from build123d import *


with BuildPart() as f2:
    # F2: sweep along a path in F1
    with BuildLine(Plane.XZ) as f2_path:
        Line((0, 0), (-0.868731, 2.386819))
    # F0 (on Top) → F2 (sweep)
    with BuildSketch(Plane.XY):
        with BuildLine():
            Line((0, 14.836045), (-1.27, 12.63634))
            ThreePointArc((-1.27, 12.63634), (-1.591732, 12.599857), (-1.912429, 12.555183))
            Line((-1.912429, 12.555183), (-3.689574, 14.369943))
            Line((-3.689574, 14.369943), (-4.372631, 11.92351))
            ThreePointArc((-4.372631, 11.92351), (-4.675182, 11.808161), (-4.974694, 11.685137))
            Line((-4.974694, 11.685137), (-7.147319, 13.000925))
            Line((-7.147319, 13.000925), (-7.200513, 10.461482))
            ThreePointArc((-7.200513, 10.461482), (-7.464873, 10.274516), (-7.72438, 10.080871))
            Line((-7.72438, 10.080871), (-10.155972, 10.815011))
            Line((-10.155972, 10.815011), (-9.57596, 8.342121))
            ThreePointArc((-9.57596, 8.342121), (-9.785518, 8.095285), (-9.988715, 7.843186))
            Line((-9.988715, 7.843186), (-12.526487, 7.94955))
            Line((-12.526487, 7.94955), (-11.349715, 5.698593))
            ThreePointArc((-11.349715, 5.698593), (-11.491304, 5.407397), (-11.625422, 5.112686))
            Line((-11.625422, 5.112686), (-14.109917, 4.58459))
            Line((-14.109917, 4.58459), (-12.410326, 2.697002))
            ThreePointArc((-12.410326, 2.697002), (-12.475048, 2.379743), (-12.531662, 2.060936))
            Line((-12.531662, 2.060936), (-14.806769, 0.931563))
            Line((-14.806769, 0.931563), (-12.691149, -0.474052))
            ThreePointArc((-12.691149, -0.474052), (-12.674939, -0.79744), (-12.65049, -1.120309))
            Line((-12.65049, -1.120309), (-14.573258, -2.779998))
            Line((-14.573258, -2.779998), (-12.174542, -3.615319))
            ThreePointArc((-12.174542, -3.615319), (-12.078418, -3.924516), (-11.974442, -4.231162))
            Line((-11.974442, -4.231162), (-13.424055, -6.316881))
            Line((-13.424055, -6.316881), (-10.892963, -6.529422))
            ThreePointArc((-10.892963, -6.529422), (-10.722965, -6.805), (-10.545996, -7.076155))
            Line((-10.545996, -7.076155), (-11.431369, -9.456851))
            Line((-11.431369, -9.456851), (-8.926939, -9.033258))
            ThreePointArc((-8.926939, -9.033258), (-8.693748, -9.257902), (-8.454906, -9.476527))
            Line((-8.454906, -9.476527), (-8.720408, -12.002613))
            Line((-8.720408, -12.002613), (-6.400003, -10.969501))
            ThreePointArc((-6.400003, -10.969501), (-6.118272, -11.129095), (-5.832563, -11.281454))
            Line((-5.832563, -11.281454), (-5.461512, -13.794206))
            Line((-5.461512, -13.794206), (-3.470931, -12.21649))
            ThreePointArc((-3.470931, -12.21649), (-3.158362, -12.301006), (-2.843739, -12.377526))
            Line((-2.843739, -12.377526), (-1.859449, -14.719058))
            Line((-1.859449, -14.719058), (-0.323768, -12.695872))
            ThreePointArc((-0.323768, -12.695872), (0, -12.7), (0.323768, -12.695872))
            Line((0.323768, -12.695872), (1.859449, -14.719058))
            Line((1.859449, -14.719058), (2.843739, -12.377526))
            ThreePointArc((2.843739, -12.377526), (3.158362, -12.301006), (3.470931, -12.21649))
            Line((3.470931, -12.21649), (5.461512, -13.794206))
            Line((5.461512, -13.794206), (5.832563, -11.281454))
            ThreePointArc((5.832563, -11.281454), (6.118272, -11.129095), (6.400003, -10.969501))
            Line((6.400003, -10.969501), (8.720408, -12.002613))
            Line((8.720408, -12.002613), (8.454906, -9.476527))
            ThreePointArc((8.454906, -9.476527), (8.693748, -9.257902), (8.926939, -9.033258))
            Line((8.926939, -9.033258), (11.431369, -9.456851))
            Line((11.431369, -9.456851), (10.545996, -7.076155))
            ThreePointArc((10.545996, -7.076155), (10.722965, -6.805), (10.892963, -6.529422))
            Line((10.892963, -6.529422), (13.424055, -6.316881))
            Line((13.424055, -6.316881), (11.974442, -4.231162))
            ThreePointArc((11.974442, -4.231162), (12.078418, -3.924516), (12.174542, -3.615319))
            Line((12.174542, -3.615319), (14.573258, -2.779998))
            Line((14.573258, -2.779998), (12.65049, -1.120309))
            ThreePointArc((12.65049, -1.120309), (12.674939, -0.79744), (12.691149, -0.474052))
            Line((12.691149, -0.474052), (14.806769, 0.931563))
            Line((14.806769, 0.931563), (12.531662, 2.060936))
            ThreePointArc((12.531662, 2.060936), (12.475048, 2.379743), (12.410326, 2.697002))
            Line((12.410326, 2.697002), (14.109917, 4.58459))
            Line((14.109917, 4.58459), (11.625422, 5.112686))
            ThreePointArc((11.625422, 5.112686), (11.491304, 5.407397), (11.349715, 5.698593))
            Line((11.349715, 5.698593), (12.526487, 7.94955))
            Line((12.526487, 7.94955), (9.988715, 7.843186))
            ThreePointArc((9.988715, 7.843186), (9.785518, 8.095285), (9.57596, 8.342121))
            Line((9.57596, 8.342121), (10.155972, 10.815011))
            Line((10.155972, 10.815011), (7.72438, 10.080871))
            ThreePointArc((7.72438, 10.080871), (7.464873, 10.274516), (7.200513, 10.461482))
            Line((7.200513, 10.461482), (7.147319, 13.000925))
            Line((7.147319, 13.000925), (4.974694, 11.685137))
            ThreePointArc((4.974694, 11.685137), (4.675182, 11.808161), (4.372631, 11.92351))
            Line((4.372631, 11.92351), (3.689574, 14.369943))
            Line((3.689574, 14.369943), (1.912429, 12.555183))
            ThreePointArc((1.912429, 12.555183), (1.591732, 12.599857), (1.27, 12.63634))
            Line((1.27, 12.63634), (0, 14.836045))
        make_face()
    sweep(path=f2_path.line)


solid = f2.part
CAD build for the part. Positions are in the model's coordinates, mm. A direction names the side the tool comes from. Give positions to 0.01 mm unless a question says otherwise; leave off trailing zeros. Write each loop counter-clockwise with the first axis right and the second up, starting at its lowest first coordinate (ties: lowest second). Pieces come first, ordered by that corner, then holes. Notation, with made-up numbers: M 70.25,-35 L 75.25,-35 A23 ccw 75.25,-16 Z; hole C -31.75,84 d7. An arc over 180 degrees is marked long. Put each result on its own line as item: value. Start each with the question number.
(1) Band-saw the part on A-A, the plane y = -10.25. Write the cut outline in (x, z).
(2) Probe L1, parallel to Y at x = -14, z = 1.9; L2, parallel to Y at x = 12.5, z = 1.7; L3, parallel to Y at x = -12, z = 0.4. List the from-to ranges inside material, lowest first.
(3) Band-saw the part on B-B, the plane y = 0. Write the cut outline in (x, z).
(4) Mould opens along X. For faces 5 (the face through (-4.466, 13.167, 1.21)), 6 (the face through (0, 0, 0)), 7 (the face through (3.596, 13.126, 1.21)), 8 (the face through (11.49, 6.81, 1.21)) say: +X half, -X half, draft (parallel to the pull), parting line (faces both ways), or undercut.
(5) Which spindle directions (+Z, -Z, +X, -X, +Y, -Y) get a long thin tool onto all of the face, cutting with end or side? Do faces 1 (the face through (-1, 0, 2.387)), 2 (the face through (5.2, -12.6, 1.2)), 3 (the face through (12.46, 4.84, 1.21)), 4 (the face through (-13.8, -3.2, 1.2)). Say none if no direction does.
(6) Flat gauge pin, fed straight in: pin 1 Ø1 at (x, y) = (8.5, -9) entering from -Z. Where does the tip first touch, or does it go through?
Response values:
1. outline: M -9.4,2.39 L -8.54,0 L 8.54,0 L 7.67,2.39 Z
2. L1: y = -6.33 to -6.15, -3.22 to -1.69, -0.06 to 1.68, 3.69 to 4.75
2. L2: y = -6.34 to -5.88, -3.29 to -1.52, -0.19 to 1.77, 3.48 to 4.8
2. L3: y = -6.45 to 5.06, 6.66 to 7.92
3. outline: M -14.27,2.39 L -13.4,0 L 13.4,0 L 12.54,2.39 Z
4. face 5: undercut
4. face 6: draft
4. face 7: undercut
4. face 8: +X half
5. face 1: +Z, +X, -X, +Y, -Y
5. face 2: +Z, -Y
5. face 3: +Z, +X
5. face 4: -Z, -X
6. pin 1: stops at z = 0
